Part model, mm, in its own coordinate system. Round coordinates to 2 decimals unless told otherwise and drop trailing zeros. Loops run counter-clockwise (first coordinate to the right, second up) from the corner with the lowest first, then second, coordinate; pieces in that order, holes last.
(1) Cut at C-C on z = 3. List the corners of the cut face in (x, y), then the cut area to 3 significant figures.
(2) Mould opens along Y. For faces 1 (the face through (2, -1, 3)), 2 (the face through (2.31, -0.96, 39.44)), 3 (the face through (0, -2, 0)) say: +Y half, -Y half, draft (parallel to the pull), parting line (faces both ways), or undercut.
(3) Flat gauge pins, fed straight in: pin 1 (1.6 mm diameter, centred on y = 0, z = 3, fed in from +X); pin 2 (1 mm diameter, centred on x = 1, z = 34, fed in from -Y). Where does each tip first touch, or does it go through?
(4) Cut at B-B on y = 0. List the corners of the cut face in (x, z).
(5) Cut at D-D on z = 63. List the corners of the cut face in (x, y).
(6) Probe probe 1 along Y at (x, z) = (0, 38.5); probe 2 along Z at (x, y) = (-2.25, 0.3). List the from-to ranges inside material, lowest first.
(7) Cut at A-A on x = 0. List the corners of the cut face in (y, z), then the cut area to 3 significant figures.
from build123d import *

# Parameters (mm, degrees)
F0_R     = 2.5
F0_R_2   = 1.5
F1_DEPTH = 80
F3_D     = 2
F3_DEPTH = 2.501
F4_D     = 2


with BuildPart() as f1:
    # F0 (on Top) → F1 (new body)
    with BuildSketch(Plane.XY):
        Circle(F0_R)
        Circle(F0_R_2, mode=Mode.SUBTRACT)
    extrude(amount=F1_DEPTH)

    # F3 (through all, one way)
    with BuildSketch(Plane.YZ):
        with Locations((0, 3)):
            Circle(F3_D / 2)
    extrude(amount=-F3_DEPTH, mode=Mode.SUBTRACT)

    # F4 (through all)
    with Locations(Plane(origin=(0, 0, 0), x_dir=(0, 1, 0), z_dir=(-1, 0, 0))):
        with Locations((0, -3)):
            Hole(F4_D / 2)


solid = f1.part
Final values:
1. outline: (-2.29, -1) arc R2.5 ccw to (2.29, -1) - (1.12, -1) arc R1.5 cw to (-1.12, -1) - close; (-2.29, 1) - (-1.12, 1) arc R1.5 cw to (1.12, 1) - (2.29, 1) arc R2.5 ccw to start
1. area: 8.36 mm2
2. face 1: undercut
2. face 2: parting line
2. face 3: draft
3. pin 1: passes through
3. pin 2: stops at y = -2.45
4. outline: (-2.5, 0) - (-1.5, 0) - (-1.5, 2) - (-2.5, 2) - close; (-2.5, 4) - (-1.5, 4) - (-1.5, 80) - (-2.5, 80) - close; (1.5, 0) - (2.5, 0) - (2.5, 2) - (1.5, 2) - close; (1.5, 4) - (2.5, 4) - (2.5, 80) - (1.5, 80) - close
5. outline: circle Ø5 at (0, 0); hole circle Ø3 at (0, 0)
6. probe 1: y = -2.5 to -1.5, 1.5 to 2.5
6. probe 2: z = 0 to 2.05, 3.95 to 80
7. outline: (-2.5, 0) - (-1.5, 0) - (-1.5, 80) - (-2.5, 80) - close; (1.5, 0) - (2.5, 0) - (2.5, 80) - (1.5, 80) - close
7. area: 160 mm2
